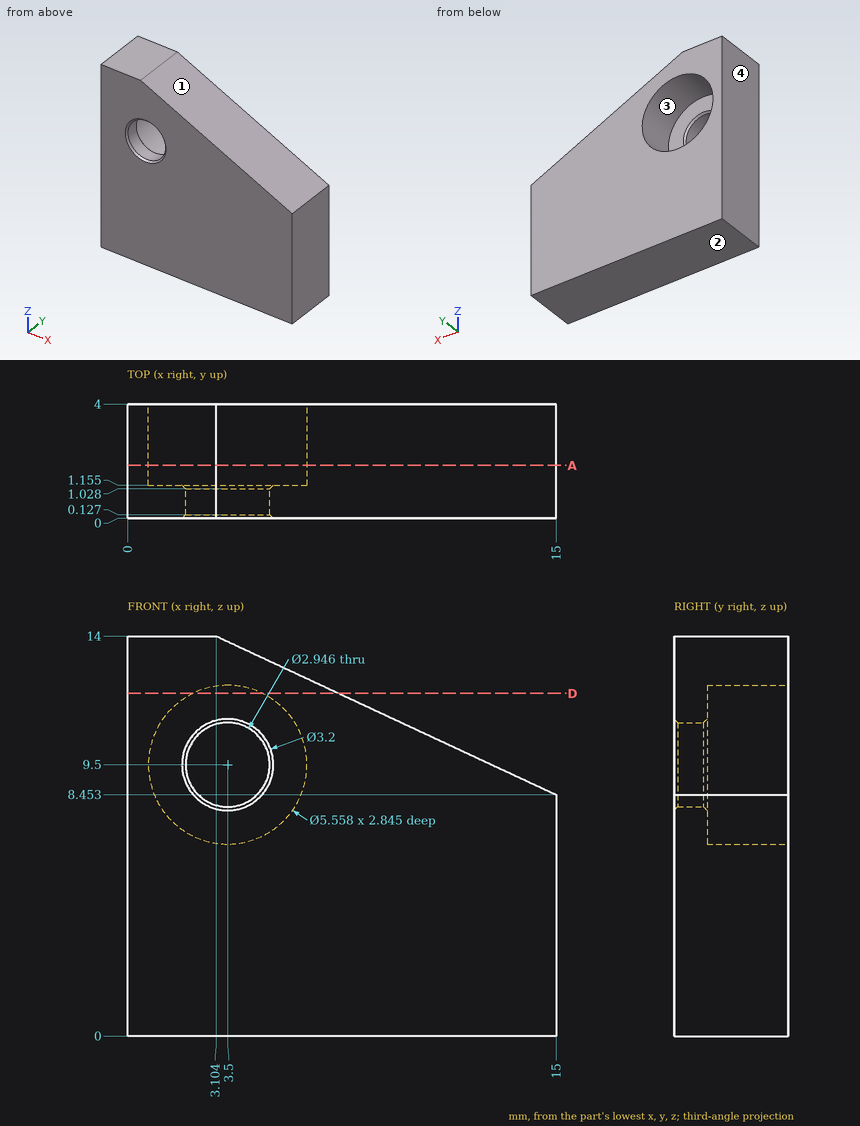
The figure shows three views and two pictorial views of one solid part (mm, origin at its lowest corner). Answer the questions. Round coordinates to 2 decimals unless told otherwise and drop trailing zeros. Order: outer loops, then holes, each group sorted by start corner. A loop starts at its lowest first (then second) coordinate and runs counter-clockwise, first axis right, second up. Notation, with made-up numbers: M -6,6.5 L 19,6.5 A19 ccw 19,41.5 Z; hole C 50,67 d9. An arc over 180 degrees is marked long. Put each result on its own line as item: value. Start each with the question number.
Q1. For a pull along X with two mould halves and no side action, classify the marked faces 1, 2, 3 and 4 as pulls with the +X half, pulls with the -X half, needs draft (parallel to the pull), parting line crosses it, or undercut.
Q2. Flat-ended cylindrical pins translate along their axes: pin 1 (1.8 mm diameter, centred on x = 3.5, z = 9.5, fed in from -Y); pin 2 (3 mm diameter, centred on x = 3.5, z = 9, fed in from +Y) (1 decimal). Find the tip coordinate at first contact, or state that the pin passes through.
Q3. Straight lines are drawn through the part: L1, parallel to Z at x = 3.5, y = 2.1 (1 decimal); L2, parallel to X at y = 3.25, z = 9 (1 decimal); L3, parallel to Y at x = 3.5, z = 11.5 (1 decimal). For each, find the intervals that lie inside material, in ascending order. Write a range as [from, to].
Q4. Section A-A, the plane y = 1.85 is taken. Write down the section's boundary in (x, z), and give its area (3 significant figures).
Q5. Section D-D, the plane z = 12 is taken. Write down the section's boundary in (x, y) (1 decimal).
Findings below:
1. face 1: pulls with the +X half
1. face 2: needs draft
1. face 3: undercut
1. face 4: pulls with the -X half
2. pin 1: passes through
2. pin 2: stops at y = 1.2
3. L1: z = [0, 6.7], [12.3, 13.8]
3. L2: x = [0, 0.8], [6.2, 13.8]
3. L3: y = [0, 1.2]
4. outline: M 0,0 L 15,0 L 15,8.45 L 3.1,14 L 0,14 Z; hole C 3.5,9.5 d5.56
4. area: 153 mm^2
5. outline: M 0,0 L 7.4,0 L 7.4,4 L 4.7,4 L 4.7,1.2 L 2.3,1.2 L 2.3,4 L 0,4 Z
